Model file for the job. Use its own axes, mm. A direction names the side the tool comes from. Coordinates: 2 decimals unless noted, no trailing zeros. Order: outer loops, then holes, each group sorted by start corner. A loop starts at its lowest first (then second) coordinate and runs counter-clockwise, first axis right, second up.
from build123d import *

# Parameters (mm, degrees)
BOSS_EXTRUDE1_DEPTH   = 150
BOSS_EXTRUDE1_2_DEPTH = 150
SKETCH2_R             = 15
BOSS_EXTRUDE2_DEPTH   = 5
SKETCH3_W             = 30
SKETCH3_H             = 63.5
BOSS_EXTRUDE3_DEPTH   = 15.24
SKETCH4_R             = 5.08
CUT_EXTRUDE1_DEPTH    = 183.315406919
CUT_EXTRUDE3_START    = -16.75
CUT_EXTRUDE3_DEPTH    = 16.75
CUT_EXTRUDE4_START    = -16.75
CUT_EXTRUDE4_DEPTH    = 16.75
SKETCH7_W             = 63.5
SKETCH7_H             = 7.62
CUT_EXTRUDE5_DEPTH    = 176.754715726
SKETCH8_W             = 30
SKETCH8_H             = 3.81
BOSS_EXTRUDE4_DEPTH   = 10
CUT_EXTRUDE6_START    = -7.62
CUT_EXTRUDE6_DEPTH    = 7.62
SKETCH1_4_R           = 1.25
CUT_EXTRUDE7_DEPTH    = 10
BOSS_EXTRUDE5_START   = 3.8
BOSS_EXTRUDE5_DEPTH   = 3.8
FILLET1_R             = 1
CUT_EXTRUDE8_REACH    = 173.256
SKETCH9_R             = 1.7


# Read off the part's stored shape, not the designer's step: Cut-Extrude6
with BuildPart() as part:
    # Sketch1 → Boss-Extrude1 (new body)
    with BuildSketch(Plane(origin=(0, 0, 0), x_dir=(1, 0, 0), z_dir=(0, 1, 0))):
        with BuildLine():
            Line((-5.75, 13.854151002), (-5.75, -13.854151002))
            ThreePointArc((-5.75, -13.854151002), (-15, 0), (-5.75, 13.854151002))
        make_face()
    extrude(amount=BOSS_EXTRUDE1_DEPTH)



with BuildPart() as body_2:
    # Sketch1 → Boss-Extrude1 2 (new body)
    with BuildSketch(Plane(origin=(0, 0, 0), x_dir=(1, 0, 0), z_dir=(0, 1, 0))):
        with BuildLine():
            Line((5.75, 13.854151002), (5.75, -13.854151002))
            ThreePointArc((5.75, -13.854151002), (15, 0), (5.75, 13.854151002))
        make_face()
    extrude(amount=BOSS_EXTRUDE1_2_DEPTH)


with BuildPart() as part_1:
    add(part.part)

    add(body_2.part)  # Boss-Extrude2 merges body 2
    # Sketch2 → Boss-Extrude2 (add)
    with BuildSketch(Plane(origin=(0, 150, 0), x_dir=(1, 0, 0), z_dir=(0, 1, 0))):
        with Locations(Location((0, 0, 0), (0, 0, 112.540310464))):
            Circle(SKETCH2_R)
    extrude(amount=BOSS_EXTRUDE2_DEPTH)

    # Sketch3 → Boss-Extrude3 (add)
    with BuildSketch(Plane(origin=(0, 155, 0), x_dir=(1, 0, 0), z_dir=(0, 1, 0))):
        Rectangle(SKETCH3_W, SKETCH3_H)
    extrude(amount=BOSS_EXTRUDE3_DEPTH)

    # Sketch4 → Cut-Extrude1 (cut, through all)
    with BuildSketch(Plane.XY.offset(31.75)):
        with Locations((0, 162.62)):
            Circle(SKETCH4_R)
    extrude(amount=-CUT_EXTRUDE1_DEPTH, mode=Mode.SUBTRACT)

    # Sketch6 → Cut-Extrude3 (cut)
    with BuildSketch(Plane(origin=(0, 0, -31.75), x_dir=(-1, 0, 0), z_dir=(0, 0, -1)).offset(CUT_EXTRUDE3_START)):
        with BuildLine():
            ThreePointArc((-9.9e-08, 170.24), (7.62, 162.62000005), (0, 155))
            Line((0, 155), (15, 155))
            Line((15, 155), (15, 170.24))
            Line((15, 170.24), (-9.9e-08, 170.24))
        make_face()
        with BuildLine():
            ThreePointArc((0, 155), (-7.62, 162.61999995), (-9.9e-08, 170.24))
            Line((-9.9e-08, 170.24), (-15, 170.24))
            Line((-15, 170.24), (-15, 155))
            Line((-15, 155), (0, 155))
        make_face()
    extrude(amount=CUT_EXTRUDE3_DEPTH, mode=Mode.SUBTRACT)

    # Sketch4<4> → Cut-Extrude4 (cut)
    with BuildSketch(Plane.XY.offset(31.75).offset(CUT_EXTRUDE4_START)):
        with BuildLine():
            ThreePointArc((-9.9e-08, 170.24), (7.62, 162.62000005), (0, 155))
            Line((0, 155), (15, 155))
            Line((15, 155), (15, 170.24))
            Line((15, 170.24), (-9.9e-08, 170.24))
        make_face()
        with BuildLine():
            ThreePointArc((0, 155), (-7.62, 162.61999995), (-9.9e-08, 170.24))
            Line((-9.9e-08, 170.24), (-15, 170.24))
            Line((-15, 170.24), (-15, 155))
            Line((-15, 155), (0, 155))
        make_face()
    extrude(amount=CUT_EXTRUDE4_DEPTH, mode=Mode.SUBTRACT)

    # Sketch7 → Cut-Extrude5 (cut, through all)
    with BuildSketch(Plane.ZY.offset(15)):
        with Locations((0, 166.43)):
            Rectangle(SKETCH7_W, SKETCH7_H)
    extrude(amount=-CUT_EXTRUDE5_DEPTH, mode=Mode.SUBTRACT)

    # Sketch8 → Boss-Extrude4 (add)
    with BuildSketch(Plane.ZY.offset(15)):
        with Locations((0, 160.715)):
            Rectangle(SKETCH8_W, SKETCH8_H)
    boss_extrude4 = extrude(amount=BOSS_EXTRUDE4_DEPTH)

    # Mirror2: Boss-Extrude4 across plane
    add(boss_extrude4.mirror(Plane(origin=(0, 0, 0), x_dir=(0, 0, 1), z_dir=(1, 0, 0))))

    # Cut-Extrude6 outline → Cut-Extrude6 (cut)
    with BuildSketch(Plane(origin=(0, 162.62, 0), x_dir=(1, 0, 0), z_dir=(0, 1, 0)).offset(CUT_EXTRUDE6_START)):
        with BuildLine():
            Line((25, 15), (10, 15))
            ThreePointArc((10, 15), (20.606601718, 10.606601718), (25, 0))
            Line((25, 0), (25, 15))
        make_face()
        with BuildLine():
            Line((25, -15), (25, 0))
            ThreePointArc((25, 0), (20.606601718, -10.606601718), (10, -15))
            Line((10, -15), (25, -15))
        make_face()
    cut_extrude6 = extrude(amount=CUT_EXTRUDE6_DEPTH, mode=Mode.SUBTRACT)

    # Mirror3: Cut-Extrude6 across plane
    add(cut_extrude6.mirror(Plane(origin=(0, 0, 0), x_dir=(0, 0, 1), z_dir=(1, 0, 0))), mode=Mode.SUBTRACT)

    # Sketch1<4> → Cut-Extrude7 (cut)
    with BuildSketch(Plane(origin=(0, 0, 0), x_dir=(1, 0, 0), z_dir=(0, 1, 0))):
        with Locations(Location((-8, 0, 0), (0, 0, 270))):
            Circle(SKETCH1_4_R)
        with Locations(Location((8, 0, 0), (0, 0, 270))):
            Circle(SKETCH1_4_R)
    extrude(amount=CUT_EXTRUDE7_DEPTH, mode=Mode.SUBTRACT)

    # Sketch12 → Boss-Extrude5 (add)
    with BuildSketch(Plane.XZ.offset(BOSS_EXTRUDE5_START)):
        with BuildLine():
            Line((-5.75, 9.669539803), (-5.75, 13.854151002))
            ThreePointArc((-5.75, 13.854151002), (-15, 0), (-5.75, -13.854151002))
            Line((-5.75, -13.854151002), (-5.75, -9.669539803))
            ThreePointArc((-5.75, -9.669539803), (-11.25, 0), (-5.75, 9.669539803))
        make_face()
        with BuildLine():
            ThreePointArc((5.75, -13.854151002), (15, 0), (5.75, 13.854151002))
            Line((5.75, 13.854151002), (5.75, 9.669539803))
            ThreePointArc((5.75, 9.669539803), (11.25, 0), (5.75, -9.669539803))
            Line((5.75, -9.669539803), (5.75, -13.854151002))
        make_face()
    extrude(amount=-BOSS_EXTRUDE5_DEPTH)

    # Fillet1
    fillet1_edges = [part_1.edges().sort_by_distance(p)[0] for p in [
        (15, 158.81, 0),
        (-15, 158.81, 0),
    ]]
    fillet(fillet1_edges, radius=FILLET1_R)

    # Sketch9 → Cut-Extrude8 (cut, up to next)
    with BuildSketch(Plane(origin=(0, 162.62, 0), x_dir=(1, 0, 0), z_dir=(0, 1, 0)), mode=Mode.PRIVATE) as cut_extrude8_sk1:
        with Locations(Location((-19.31, 0, 0), (0, 0, 270))):
            Circle(SKETCH9_R)
    cut_extrude8_tool1 = extrude(cut_extrude8_sk1.sketch, amount=-CUT_EXTRUDE8_REACH, mode=Mode.PRIVATE) & part_1.part
    # Sketch9 → Cut-Extrude8 (cut, up to next)
    with BuildSketch(Plane(origin=(0, 162.62, 0), x_dir=(1, 0, 0), z_dir=(0, 1, 0)), mode=Mode.PRIVATE) as cut_extrude8_sk2:
        with Locations(Location((19.31, 0, 0), (0, 0, 270))):
            Circle(SKETCH9_R)
    cut_extrude8_tool2 = extrude(cut_extrude8_sk2.sketch, amount=-CUT_EXTRUDE8_REACH, mode=Mode.PRIVATE) & part_1.part
    add(cut_extrude8_tool1.solids().sort_by_distance((-19.31, 162.62, 0))[0], mode=Mode.SUBTRACT)
    add(cut_extrude8_tool2.solids().sort_by_distance((19.31, 162.62, 0))[0], mode=Mode.SUBTRACT)


solid = part_1.part
Q1. Probe line 1 (X direction, y = 4.5, z = 0); line 2 (Y direction, x = -6, z = 2.5); line 3 (Z direction, x = 6, y = 28). List the from-to ranges inside material, lowest first.
Established:
line 1: x = -15 to -9.25, -6.75 to -5.75, 5.75 to 6.75, 9.25 to 15
line 2: y = 0 to 162.62
line 3: z = -13.75 to 13.75
Q2. Cut at B-B, the plane z = -11.5. List the corners of the cut face in (x, y), plus the area to 3 significant figures.
Established:
outline: (-19.63, 158.81) - (-16, 158.81) arc R1 cw to (-15, 157.81) - (-15, 155) - (-9.63, 155) - (-9.63, -3.8) - (-5.75, -3.8) - (-5.75, 150) - (5.75, 150) - (5.75, -3.8) - (9.63, -3.8) - (9.63, 155) - (15, 155) - (15, 157.81) arc R1 cw to (16, 158.81) - (19.63, 158.81) - (19.63, 162.62) - (5.08, 162.62) arc R5.08 cw to (-5.08, 162.62) - (-19.63, 162.62) - close
area: 1,510 mm2
Q3. Drop flat-ended pins along their axis: P1, Ø2.5, axis at x = 18.5, z = -0.5, coming from the -Y side; P2, Ø5, axis at y = 22, z = -16.5, coming from the -X side; P3, Ø4, axis at x = -8, z = 0, coming from the -Y side; P4, Ø1.5, axis at y = 102, z = -7.5, coming from the -X side. Give the stop position or say it passes through.
Established:
P1: stops at y = 158.81
P2: passes through
P3: stops at y = 0
P4: stops at x = -13.4
Q4. Which spindle directions (+Z, -Z, +X, -X, +Y, -Y) get a long thin tool onto all of the face, cutting with end or side? Do faces 1 (the face through (6.6, 0, -0.1)), 2 (the face through (11, 155, 11)), 3 (the face through (-21.4, 158.81, -0.2)), 4 (the face through (11, 155, -12)). Say none if no direction does.
Established:
face 1: -Y
face 2: +Z, +X, -Y
face 3: +Z, -Z, -X, -Y
face 4: -Z, +X, -Y
Q5. Mould opens along Z. For faces 5 (the face through (-6.6, 0, -0.1)), 6 (the face through (7, 158, -15)), 7 (the face through (-11, 155, -11)) say: pulls with the +Z half, pulls with the -Z half, needs draft (parallel to the pull), parting line crosses it, or undercut.
Established:
face 5: undercut
face 6: pulls with the -Z half
face 7: needs draft
Q6. Cut at C-C, the plane z = 23.5. List the corners of the cut face in (x, y), plus the area to 3 significant figures.
Established:
outline: (-7.62, 162.62) arc R7.62 ccw to (7.62, 162.62) - (5.08, 162.62) arc R5.08 cw to (-5.08, 162.62) - close
area: 50.7 mm2
Q7. Cut at A-A, the plane y = 84. List the corners of the cut face in (x, z).
Established:
outline: (-5.75, -13.85) - (-5.75, 13.85) arc R15 ccw to start; (5.75, -13.85) arc R15 ccw to (5.75, 13.85) - close
